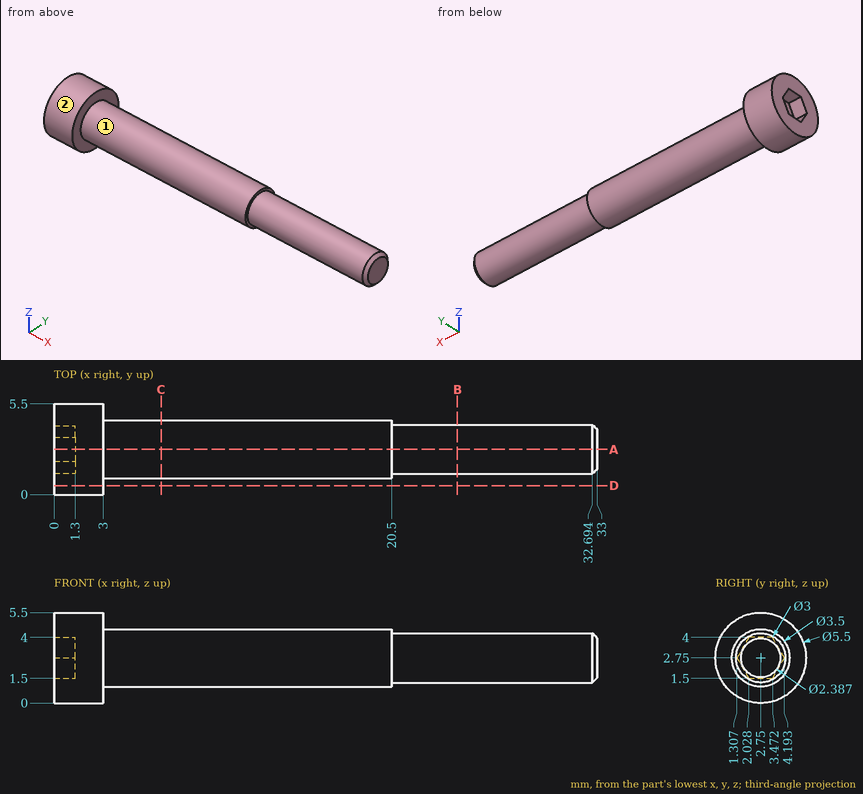
Source: three-view drawing plus pictorial views. Frame: mm from the lowest corner of the part. A direction names the side the tool comes from. Round coordinates to 2 decimals unless told otherwise and drop trailing zeros. Order: outer loops, then holes, each group sorted by start corner. A loop starts at its lowest first (then second) coordinate and runs counter-clockwise, first axis right, second up. Notation, with made-up numbers: (20.5, 79) - (64.5, 79) arc R26 cw to (64.5, 103) - close; hole circle Ø5 at (26, 7). An arc over 180 degrees is marked (long way). Write each question's results on one line, items separated by ' | '.
Item 1: First-contact query: pin 1 Ø1 at (y, z) = (2, 4.5) entering from +X; pin 2 Ø1.5 at (x, z) = (21, 3.5) entering from +Y; pin 3 Ø3 at (x, z) = (11, 3.5) entering from -Y. Flat tips, straight axial feed; report the tip coordinate or a pass-through.
Completed:
pin 1: x = 32.79 | pin 2: y = 4.49 | pin 3: y = 1
Item 2: Reachability of the marked faces 1 and 2 from +Z, -Z, +X, -X, +Y, -Y: full face, straight path, thin tool, end or side. Return the list, or none.
Completed:
face 1: +X | face 2: +X, -X
Item 3: Material intervals for line 1 along X through (y, z) = (1.3, 0.65); line 2 along X through (y, z) = (2.7, 2.6); line 3 along Y through (x, z) = (22.5, 4.05) (1 decimal), sorted ascending. Write a range as [from, to].
Completed:
line 1: [0, 3] | line 2: [1.3, 33] | line 3: [2, 3.5]
Item 4: Section B-B, the plane x = 24.5. Return the cut outline in (y, z).
Completed:
outline: circle Ø3 at (2.75, 2.75)
Item 5: Section A-A, the plane y = 2.75. Return the cut outline in (x, z).
Completed:
outline: (0, 0) - (3, 0) - (3, 1) - (20.5, 1) - (20.5, 1.25) - (32.69, 1.25) - (33, 1.56) - (33, 3.94) - (32.69, 4.25) - (20.5, 4.25) - (20.5, 4.5) - (3, 4.5) - (3, 5.5) - (0, 5.5) - (0, 4) - (1.3, 4) - (1.3, 1.5) - (0, 1.5) - close
Item 6: Section C-C, the plane x = 6.5. Return the cut outline in (y, z).
Completed:
outline: circle Ø3.5 at (2.75, 2.75)
Item 7: Section D-D, the plane y = 0.55. Return the cut outline in (x, z).
Completed:
outline: (0, 1.1) - (3, 1.1) - (3, 4.4) - (0, 4.4) - close
